Source: CAD feature listing. Evaluate the final solid. Frame: model axes, mm. Face numbers are marked on the shaded views. A direction names the side the tool comes from. Coordinates: 2 decimals unless noted, no trailing zeros. Order: outer loops, then holes, each group sorted by start corner. A loop starts at its lowest first (then second) coordinate and runs counter-clockwise, first axis right, second up. Notation, with made-up numbers: (-25, -40) -> (10, -40) arc R27 cw to (10, -19) -> close; hole circle Ø5 at (6.25, 65). An arc over 180 degrees is marked (long way). Write item = value, one per line. Start each with the question number.
Item 1: Set-up query: the marked faces 4 and 5. Return all of +Z, -Z, +X, -X, +Y, -Y with unobstructed straight access to the full face (end or side cutting, diameter ignored); none if empty.
Item 2: Section query A-A (x = 0). Output: boundary loops of the cut face in (y, z).
Item 3: Ray query, line 1 along Z through (x, y) = (5, 0.5); line 2 along X through (y, z) = (-1.5, -4); line 3 along X through (y, z) = (-2, -1.5). Return the intervals inside material, ascending. Write a range as [from, to].
Item 4: Section query C-C (z = -5). Output: boundary loops of the cut face in (x, y).
Item 5: Mould query, pull axis Y, two halves, no side actions, for the marked faces 1, 2 and 3. Classes: released by +Y, released by -Y, zero draft, split by the parting line, or undercut.
Item 6: Section query B-B (y = 0). Output: boundary loops of the cut face in (x, z), then the cut area to 3 significant figures.
Item 7: Contact query for flat-ended pins moving along their axis: pin 1 (4 mm diameter, centred on y = -1, z = -4, fed in from -X); pin 2 (1.5 mm diameter, centred on x = 0.5, y = 0, fed in from +Z); pin 3 (1 mm diameter, centred on y = 2, z = -0.5, fed in from +X). Output: stop coordinate, or through.
```python
from build123d import *

# Parameters (mm, degrees)
F2_SIZE  = 0.3
F4_R     = 2.5
F5_DEPTH = 8


# Not quite as in the source:
# - a fillet or chamfer that OpenCascade refuses, or shapes differently, is made with other operations: its cross-section is extruded or revolved along the edge and cut away or added


with BuildPart() as f1:
    # F0 (on Right) → F1 (revolve)
    with BuildSketch(Plane.YZ):
        with BuildLine():
            Line((4.25, -6.8), (4.25, -3))
            ThreePointArc((4.25, -3), (4.878497412, -1.1651468819), (6.5, -0.1009926077))
            Line((6.5, -0.1009926077), (6.5, 1))
            Line((6.5, 1), (0, 1))
            Line((0, 1), (0, 0))
            Line((0, 0), (0, -7.5))
            Line((0, -7.5), (4.25, -7.5))
            Line((4.25, -7.5), (5.1640063768, -6.9207987711))
            Line((5.1640063768, -6.9207987711), (5.1465752283, -6.7215598315))
            Line((5.1465752283, -6.7215598315), (4.25, -6.8))
        make_face()
    revolve(axis=Axis((0, 0, -3.75), (0, 0, -1)))

    # F2
    f2_edges = [f1.edges().sort_by_distance(p)[0] for p in [
        (0, -4.25, -7.5),
    ]]
    chamfer(f2_edges, length=F2_SIZE)

    # F3: fillet of radius 2 on 1 edges, made by hand

    # F3_s1 → F3_t2 (revolve, cut)
    with BuildSketch(Plane.YZ):
        with BuildLine():
            ThreePointArc((6.5, -0.1009926077), (5.7627250062, 0.702647172), (4.7134430575, 1))
            Line((4.7134430575, 1), (6.5, 1))
            Line((6.5, 1), (6.5, -0.1009926077))
        make_face()
    revolve(axis=Axis((0, 0, 1), (0, 0, -1)), mode=Mode.SUBTRACT)

    # F4 (on face) → F5 (cut)
    with BuildSketch(Plane.XY.offset(1)):
        with Locations((0, -0.2312049229)):
            Circle(F4_R)
    extrude(amount=-F5_DEPTH, mode=Mode.SUBTRACT)


solid = f1.part
```
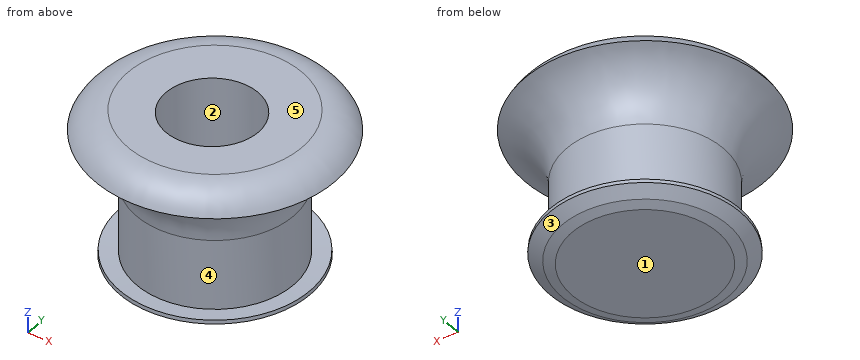
Computed:
q1.face_4 = none
q1.face_5 = +Z, +X, -X, +Y, -Y
q2.outline = (-6.5, -0.1) arc R2.99 cw to (-4.25, -3) -> (-4.25, -6.8) -> (-5.15, -6.72) -> (-5.16, -6.92) -> (-4.5, -7.34) -> (-3.95, -7.5) -> (3.95, -7.5) -> (4.5, -7.34) -> (5.16, -6.92) -> (5.15, -6.72) -> (4.25, -6.8) -> (4.25, -3) arc R2.99 cw to (6.5, -0.1) arc R2 ccw to (4.71, 1) -> (2.27, 1) -> (2.27, -7) -> (-2.73, -7) -> (-2.73, 1) -> (-4.71, 1) arc R2 ccw to start
q3.line_1 = [-7.01, -6.73], [-0.99, 0.98]
q3.line_2 = [-3.98, -2.15], [2.15, 3.98]
q3.line_3 = [-4.2, -1.77], [1.77, 4.2]
q4.outline = circle Ø8.5 at (0, 0); hole circle Ø5 at (0, -0.23)
q5.face_1 = zero draft
q5.face_2 = undercut
q5.face_3 = split by the parting line
q6.outline = (-6.5, -0.1) arc R2.99 cw to (-4.25, -3) -> (-4.25, -6.8) -> (-5.15, -6.72) -> (-5.16, -6.92) -> (-4.5, -7.34) -> (-3.95, -7.5) -> (3.95, -7.5) -> (4.5, -7.34) -> (5.16, -6.92) -> (5.15, -6.72) -> (4.25, -6.8) -> (4.25, -3) arc R2.99 cw to (6.5, -0.1) arc R2 ccw to (4.71, 1) -> (2.49, 1) -> (2.49, -7) -> (-2.49, -7) -> (-2.49, 1) -> (-4.71, 1) arc R2 ccw to start
q6.area = 40.4 mm^2
q7.pin_1 = -4.37
q7.pin_2 = -7
q7.pin_3 = 6.27
